Autodesk Inventor part; units mm, degrees
ref_plane "YZ Plane" through (0, 0, 0) normal (1, 0, 0) x (0, 1, 0)
ref_plane "XZ Plane" through (0, 0, 0) normal (0, 1, 0) x (-1, 0, 0)
ref_plane "XY Plane" through (0, 0, 0) normal (0, 0, 1) x (1, 0, 0)
sketch "Sketch1" plane through (0, 0, 0) normal (0, 0, 1) x (1, 0, 0)
  line L0 (0, 0) -> (-63.5, 0)
  line L1 (-63.5, 0) -> (-63.5, 63.5)
  line L2 (-63.5, 63.5) -> (0, 63.5)
  line L3 (0, 63.5) -> (0, 0)
  dimension "d0" = 63.5
  dimension "d1" = 63.5
extrude "Extrusion1" add sketch "Sketch1" along normal blind 96.647
sketch "Sketch2" plane through (0, 0, 0) normal (0, 0, -1) x (-1, 0, 0)
  line L0 (0, 0) -> (63.5, 0)
  line L1 (0, 63.5) -> (0, 0)
  circle A0 centre (31.75, 31.75) radius 6.35
  dimension "d4" = 12.7
  dimension "d5" = 31.75
  dimension "d6" = 31.75
extrude "Extrusion2" add sketch "Sketch2" along normal blind 88.9
sketch "Sketch3" plane through (0, 0, 96.647) normal (0, 0, 1) x (1, 0, 0)
  line L0 (-63.5, 0) -> (0, 0)
  line L1 (0, 63.5) -> (-63.5, 63.5)
  line L2 (-31.75, 63.5) -> (-31.75, 0)
  circle A0 centre (-31.75, 31.75) radius 5
  dimension "d9" = 63.5
  dimension "d10" = 10
extrude "Extrusion3" cut sketch "Sketch3" against normal blind 88.9
properties part number "p80 space thing"
Can you work these out from the model? Positions are in its coordinate system, mm. A direction names the side the tool comes from. Round coordinates to 2 decimals unless told otherwise and drop trailing zeros. Order: outer loops, then holes, each group sorted by start corner. A loop starts at its lowest first (then second) coordinate and runs counter-clockwise, first axis right, second up. Notation, with made-up numbers: (81, 7.25) - (102, 7.25) arc R33 cw to (102, 38.25) - close; hole circle Ø3 at (13, -33.5). An arc over 180 degrees is marked (long way). Answer in a Markdown table with one row per item.
(1) Which directions (+Z, -Z, +X, -X, +Y, -Y) give clear straight access to the entire face, cutting with the end or side of a thin tool? Please do faces 4 (the face through (-32, 32, 7.747)), 5 (the face through (-32, 32, -88.9)), 6 (the face through (-37.807, 29.843, -43.828)).
From the geometry:
| item | result |
|---|---|
| face 4 | +Z |
| face 5 | -Z, +X, -X, +Y, -Y |
| face 6 | -Z |
(2) Suppose I cut it at A-A, the plane z = 59. Please give me the cut outline in (x, y), plus the area to 3 significant figures.
From the geometry:
| item | result |
|---|---|
| outline | (-63.5, 0) - (0, 0) - (0, 63.5) - (-63.5, 63.5) - close; hole circle Ø10 at (-31.75, 31.75) |
| area | 3,950 mm2 |
(3) Suppose I cut it at C-C, the plane y = 31.75. Please give me the cut outline in (x, z), plus the area to 3 significant figures.
From the geometry:
| item | result |
|---|---|
| outline | (-63.5, 0) - (-38.1, 0) - (-38.1, -88.9) - (-25.4, -88.9) - (-25.4, 0) - (0, 0) - (0, 96.65) - (-26.75, 96.65) - (-26.75, 7.75) - (-36.75, 7.75) - (-36.75, 96.65) - (-63.5, 96.65) - close |
| area | 6,380 mm2 |
(4) Suppose I cut it at B-B, the plane x = -31.75. Please give me the cut outline in (y, z), plus the area to 3 significant figures.
From the geometry:
| item | result |
|---|---|
| outline | (0, 0) - (25.4, 0) - (25.4, -88.9) - (38.1, -88.9) - (38.1, 0) - (63.5, 0) - (63.5, 96.65) - (36.75, 96.65) - (36.75, 7.75) - (26.75, 7.75) - (26.75, 96.65) - (0, 96.65) - close |
| area | 6,380 mm2 |
(5) If we mould it in two halves opening along X, with no side actions, what happens to faces 1 (the face through (-39, 32, 96.647)), 2 (the face through (-63.5, 31, 48)), 3 (the face through (-35.72, 28.71, 52.82))? For each: released by +X, released by -X, zero draft, split by the parting line, or undercut.
From the geometry:
| item | result |
|---|---|
| face 1 | zero draft |
| face 2 | released by -X |
| face 3 | undercut |
(6) Suppose I cut it at D-D, the plane z = -23. Please give me the cut outline in (x, y).
From the geometry:
| item | result |
|---|---|
| outline | circle Ø12.7 at (-31.75, 31.75) |
(7) Please list where these lines run through material, in increasing order: L1, parallel to Y at x = -31.75, z = 65; L2, parallel to X at y = 31.75, z = 54; L3, parallel to Z at x = -8.5, y = 11. Write a range as from..to.
From the geometry:
| item | result |
|---|---|
| L1 | y = 0..26.75, 36.75..63.5 |
| L2 | x = -63.5..-36.75, -26.75..0 |
| L3 | z = 0..96.65 |
(8) For P1, Ø8, axis at x = -26.5, z = -49.5, coming from the -Y side; P2, Ø10, axis at y = 14.5, z = 67, coming from the +X side; P3, Ø10, axis at y = 27.5, z = -22, coming from the +X side, each with a flat end and sliding along its axis, tell me the tip position at first contact or that it passes through.
From the geometry:
| item | result |
|---|---|
| P1 | stops at y = 25.52 |
| P2 | stops at x = 0 |
| P3 | stops at x = -25.4 |
